Study the drawing (mm; zero at the part's minimum x, y, z) and answer. A direction names the side the tool comes from. Round coordinates to 2 decimals unless told otherwise and drop trailing zeros. Write each loop counter-clockwise with the first axis right and the second up, starting at its lowest first coordinate (ties: lowest second). Pieces come first, ordered by that corner, then holes.
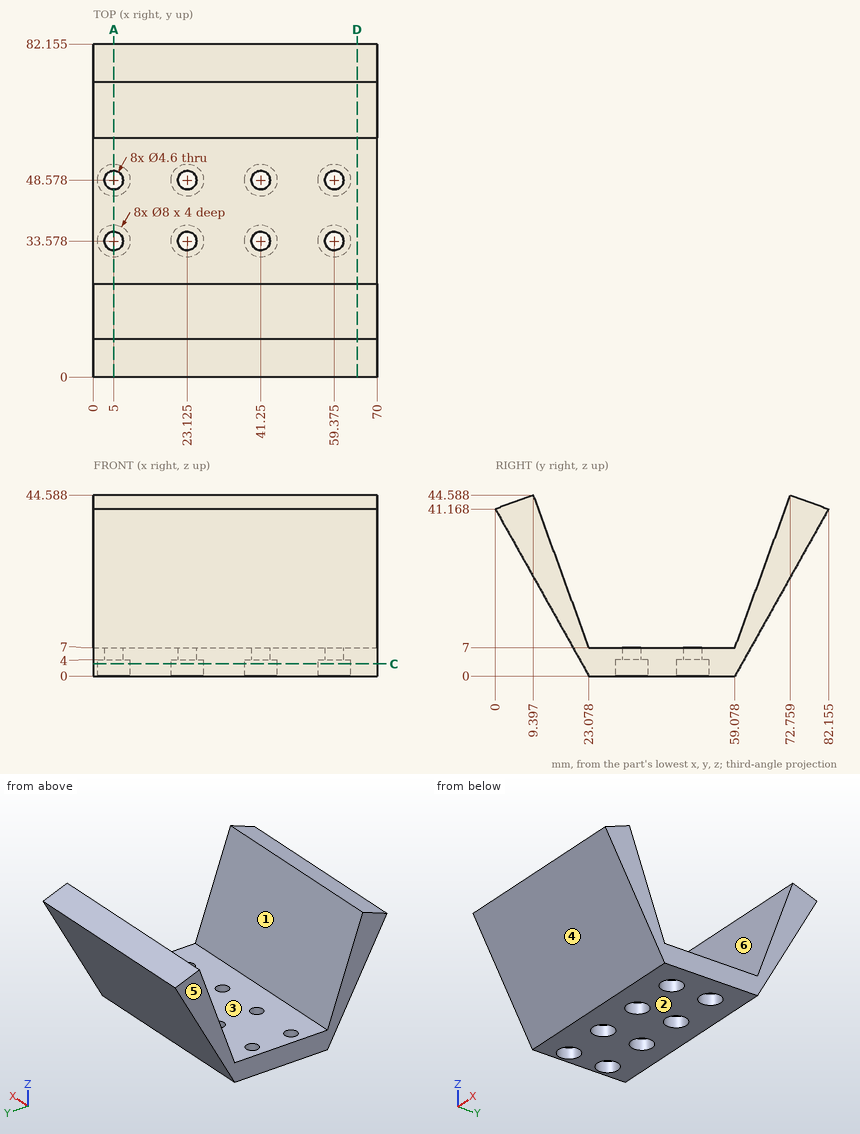
Q1. Find section D-D (x = 65). Determine the outline of the cut face in (y, z) (1 decimal).
Q2. Given pin 1 (6.5 mm diameter, centred on x = 23.12, y = 48.58, fed in from +Z); pin 2 (6 mm diameter, centred on x = 23.12, y = 48.58, fed in from -Z); pin 3 (3 mm diameter, centred on x = 59.38, y = 48.58, fed in from -Z); pin 4 (1 mm diameter, centred on x = 42, z = 40, fed in from +Y), each flat-ended and moving along its own axis, determine where each tip first touches the part or whether it passes through.
Q3. A tool of negligible diameter and unlimited length cuts with its end or side. For the marked faces 5 and 6, from which of +Z, -Z, +X, -X, +Y, -Y can it reach the whole face along a straight path? Write none if from no direction.
Q4. Find section C-C (z = 3). Count the separate pieces of the cut face and the enclosed holes in it, plus the area to 3 significant figures.
Q5. The mould has two halves that part along Y. Classify the marked faces 1, 2, 3 and 4: +Y half, -Y half, draft (parallel to the pull), parting line (faces both ways), or undercut.
Q6. Find the intervals of material crossed by L1, parallel to Y at x = 5, z = 3.1 (1 decimal); L2, parallel to Y at x = 5, z = 6.4 (1 decimal); L3, parallel to Z at x = 56.5, y = 23.5, in increasing order.
Q7. Find section A-A (x = 5). Determine the outline of the cut face in (y, z) (1 decimal).
Report:
1. outline: (0, 41.2) - (23.1, 0) - (59.1, 0) - (82.2, 41.2) - (72.8, 44.6) - (59.1, 7) - (23.1, 7) - (9.4, 44.6) - close
2. pin 1: stops at z = 7
2. pin 2: stops at z = 4
2. pin 3: passes through
2. pin 4: stops at y = 81.78
3. face 5: +Z, -Z, -X, +Y, -Y
3. face 6: +Z, +X, -X
4. separate pieces: 1
4. enclosed holes: 8
4. area: 2,350 mm2
5. face 1: undercut
5. face 2: draft
5. face 3: undercut
5. face 4: -Y half
6. L1: y = 21.3 to 29.6, 37.6 to 44.6, 52.6 to 60.8
6. L2: y = 19.5 to 31.3, 35.9 to 46.3, 50.9 to 62.7
6. L3: z = 0 to 7
7. outline: (0, 41.2) - (23.1, 0) - (29.6, 0) - (29.6, 4) - (31.3, 4) - (31.3, 7) - (23.1, 7) - (9.4, 44.6) - close; (35.9, 4) - (37.6, 4) - (37.6, 0) - (44.6, 0) - (44.6, 4) - (46.3, 4) - (46.3, 7) - (35.9, 7) - close; (50.9, 4) - (52.6, 4) - (52.6, 0) - (59.1, 0) - (82.2, 41.2) - (72.8, 44.6) - (59.1, 7) - (50.9, 7) - close
